Source: CAD feature listing. Evaluate the final solid. Frame: model axes, mm. A direction names the side the tool comes from. Give positions to 0.01 mm unless a question says otherwise; leave off trailing zeros. Loops run counter-clockwise (first coordinate to the right, second up) from the corner with the lowest first, then second, coordinate; pieces in that order, holes last. Notation, with made-up numbers: (59, 67.5) -> (110, 67.5) arc R29 ccw to (110, 91.5) -> close; hole circle Ø5 at (54, 51.5). An arc over 180 degrees is marked (long way). Return JSON: item names as keys, results as strings. Group by question number.
(1) Cut plane C-C on y = -5. Return loops of the section in (x, z).
(2) Access query for faces 1 (the face through (2.155, 1.267, -3.012)), 2 (the face through (2, -2, -4.4)). Directions: +Z, -Z, +X, -X, +Y, -Y. A direction counts if a zero-diameter tool reaches every point of the face in a straight line with its end or side. Return the directions, or none.
(3) Ray query, line 1 (Y direction, x = 0, z = 46.5); line 2 (Z direction, x = -1.75, y = -1.75); line 3 (Z direction, x = -3, y = -5.5). Return the intervals inside material, ascending. Write a range as from..to.
(4) Cut plane B-B on z = 31.5. Return loops of the section in (x, y).
(5) Cut plane A-A on x = 0. Return loops of the section in (y, z), then the cut area to 3 significant figures.
(6) Draft query along Y for faces 3 (the face through (3, -3, 0)), 4 (the face through (0.867, -3.905, 30.172)), 5 (the face through (-2.175, 1.233, -3.012)). Return one class per face: released by +Y, released by -Y, zero draft, split by the parting line, or undercut.
(7) Pin query (flat end, axial travel): pin 1 (3 mm diameter, centred on x = -4.5, z = 46, fed in from +Y); pin 2 (1.5 mm diameter, centred on y = 3, z = 14.5, fed in from -X); pin 3 (2.5 mm diameter, centred on x = 0, y = 0, fed in from -Z); pin 4 (8 mm diameter, centred on x = -2.5, y = -5, fed in from -Z). Return the tip coordinate at first contact, or that it passes through.
(8) Cut plane D-D on x = -5.75. Return loops of the section in (y, z), then the cut area to 3 significant figures.
```python
from build123d import *

# Parameters (mm, degrees)
HEX_2_DEPTH = 2.816


with BuildPart() as part:
    # sk3 → br (revolve)
    with BuildSketch(Plane(origin=(0, 0, 0), x_dir=(0, 0, -1), z_dir=(1, 0, 0)), mode=Mode.PRIVATE) as br_sk:
        Polygon((-62, 3.2), (-61.2, 4), (0, 4), (0, 0), (-62, 0), align=None)
    revolve(br_sk.sketch.rotate(Axis((0, 0, 0), (0, 0, -1)), 270), axis=Axis((0, 0, 0), (0, 0, -1)))  # turned: the seam where the file's is

    # sk1 → hd (revolve)
    with BuildSketch(Plane.ZY, mode=Mode.PRIVATE) as hd_sk:
        with BuildLine():
            Line((0, 0), (0, 7))
            Line((0, 7), (-0.88, 7))
            ThreePointArc((-0.88, 7), (-2.92552474, 5.53715631), (-4.4, 3.5))
            Line((-4.4, 3.5), (-4.4, 0))
            Line((-4.4, 0), (0, 0))
        make_face()
    revolve(hd_sk.sketch.rotate(Axis((0, 0, 0), (0, 0, -1)), 270), axis=Axis((0, 0, 0), (0, 0, -1)))  # turned: the seam where the file's is

    # sk2 → hex 2 (cut)
    with BuildSketch(Plane(origin=(0, 0, -4.4), x_dir=(-1, 0, 0), z_dir=(0, 0, -1))):
        Polygon((1.443375673, 2.5), (-1.443375673, 2.5), (-2.886751346, 0), (-1.443375673, -2.5), (1.443375673, -2.5), (2.886751346, 0), align=None)
    extrude(amount=-HEX_2_DEPTH, mode=Mode.SUBTRACT)


solid = part.part
```
Answers:
{
 "1": {"outline": "(-4.9, -0.88) arc R6 ccw to (4.9, -0.88) -> (4.9, 0) -> (-4.9, 0) -> close"},
 "2": {"face 1": "-Z", "face 2": "-Z, +X, -X, +Y, -Y"},
 "3": {"line 1": "-4..4", "line 2": "-1.58..62", "line 3": "-2.08..0"},
 "4": {"outline": "circle Ø8 at (0, 0)"},
 "5": {"outline": "(-7, -0.88) arc R7.81 ccw to (-3.5, -4.4) -> (-2.5, -4.4) -> (-2.5, -1.58) -> (2.5, -1.58) -> (2.5, -4.4) -> (3.5, -4.4) arc R7.81 ccw to (7, -0.88) -> (7, 0) -> (4, 0) -> (4, 61.2) -> (3.2, 62) -> (-3.2, 62) -> (-4, 61.2) -> (-4, 0) -> (-7, 0) -> close", "area": "533 mm²"},
 "6": {"face 3": "zero draft", "face 4": "split by the parting line", "face 5": "undercut"},
 "7": {"pin 1": "y = 2.65", "pin 2": "x = -3.31", "pin 3": "z = -1.58", "pin 4": "z = -4.4"},
 "8": {"outline": "(-3.99, -0.88) arc R5.28 ccw to (3.99, -0.88) -> (3.99, 0) -> (-3.99, 0) -> close", "area": "17.1 mm²"}
}
